from build123d import *

# Parameters (mm, degrees)
SKETCH1_R               = 14.8
BOSS_EXTRUDE1_DEPTH     = 14
SKETCH2_R               = 1.2
CUT_EXTRUDE1_DEPTH      = 1
CUT_EXTRUDE1_DEPTH_BACK = 15
SKETCH3_R               = 5.5
CUT_EXTRUDE2_DEPTH      = 14
CUT_EXTRUDE3_START      = -9
SKETCH5_R               = 2.5
CUT_EXTRUDE3_DEPTH      = 6


with BuildPart() as part:
    # Sketch1 → Boss-Extrude1 (new body)
    with BuildSketch(Plane(origin=(0, 0, 0), x_dir=(0, 0, -1), z_dir=(1, 0, 0))):
        Circle(SKETCH1_R)
    extrude(amount=BOSS_EXTRUDE1_DEPTH)

    # Sketch2 → Cut-Extrude1 (cut, two sides)
    with BuildSketch(Plane(origin=(14, 0, 0), x_dir=(0, 0, -1), z_dir=(1, 0, 0))) as cut_extrude1_sk:
        with Locations((0, 11)):
            Circle(SKETCH2_R)
        with Locations((7.778174593, 7.778174593)):
            Circle(SKETCH2_R)
        with Locations((11, 0)):
            Circle(SKETCH2_R)
        with Locations((7.778174593, -7.778174593)):
            Circle(SKETCH2_R)
        with Locations((0, -11)):
            Circle(SKETCH2_R)
        with Locations((-7.778174593, -7.778174593)):
            Circle(SKETCH2_R)
        with Locations((-11, 0)):
            Circle(SKETCH2_R)
        with Locations((-7.778174593, 7.778174593)):
            Circle(SKETCH2_R)
    extrude(amount=CUT_EXTRUDE1_DEPTH, mode=Mode.SUBTRACT)
    extrude(cut_extrude1_sk.sketch, amount=-CUT_EXTRUDE1_DEPTH_BACK, mode=Mode.SUBTRACT)

    # Sketch3 → Cut-Extrude2 (cut)
    with BuildSketch(Plane.ZY):
        Circle(SKETCH3_R)
    extrude(amount=-CUT_EXTRUDE2_DEPTH, mode=Mode.SUBTRACT)

    # Sketch5 → Cut-Extrude3 (cut, through all)
    with BuildSketch(Plane(origin=(14, 0, 0), x_dir=(0, 0, -1), z_dir=(1, 0, 0)).offset(CUT_EXTRUDE3_START)):
        with Locations((7.778174593, 7.778174593)):
            Circle(SKETCH5_R)
        with Locations((-7.778174593, -7.778174593)):
            Circle(SKETCH5_R)
        with Locations((7.778174593, -7.778174593)):
            Circle(SKETCH5_R)
        with Locations((-7.778174593, 7.778174593)):
            Circle(SKETCH5_R)
    extrude(amount=-CUT_EXTRUDE3_DEPTH, mode=Mode.SUBTRACT)


solid = part.part
Can you work these out from the model? Positions are in its coordinate system, mm. A direction names the side the tool comes from. Coordinates: 2 decimals unless noted, no trailing zeros. Loops run counter-clockwise (first coordinate to the right, second up) from the corner with the lowest first, then second, coordinate; pieces in that order, holes last. Notation, with made-up numbers: (61, -3.5) - (89, -3.5) arc R15 cw to (89, 21.5) - close; hole circle Ø9 at (-9.75, 3.25). An arc over 180 degrees is marked (long way). Answer as a JSON object with one key per item and string values. Group by question number.
Item 1: For pin 1 (14.5 mm diameter, centred on y = 0, z = 0, fed in from +X); pin 2 (3 mm diameter, centred on x = 8, y = 2, fed in from -Z); pin 3 (3 mm diameter, centred on y = -7.78, z = 7.78, fed in from -X); pin 4 (1.5 mm diameter, centred on x = 8.5, y = 3.5, fed in from -Z), each with a flat end and sliding along its axis, tell me the tip position at first contact or that it passes through.
Item 2: If we mould it in two halves opening along Y, with no side actions, what happens to faces 3 (the face through (7.098, 0.36, 9.855)), 4 (the face through (7.1, -12.17, 0.26)), 5 (the face through (6.902, -14.448, 3.208)), 6 (the face through (0, -6, 0))? For each: released by +Y, released by -Y, zero draft, split by the parting line, or undercut.
Item 3: If we section it at C-C (z = -8): List the corners of the cut face in (x, y) for me, plus the area to 3 significant figures.
Item 4: If I drill on L1, parallel to Y at x = 6, z = 0; L2, parallel to Z at x = 2.25, y = -1; L3, parallel to Z at x = 5.5, y = 0.75, over which ranges is the centre line in solid material (lowest first)? Write a range as from..to.
Item 5: If we section it at A-A (y = 0): List the corners of the cut face in (x, z) for me, plus the area to 3 significant figures.
Item 6: On a 3-axis mill with a long thin cutter (end or side, diameter ignored), from which of +Z, -Z, +X, -X, +Y, -Y can I reach the whole of each face in a straight line? I mean faces 1 (the face through (2.54, -9.3, 9.76)), 2 (the face through (14, -6, 0)). Say none if no direction works.
Item 7: If we section it at D-D (x = 4.25): State how many separate pieces and enclosed holes the cut face has, plus the area to 3 significant figures.
Returned:
{
 "1": {"pin 1": "stops at x = 14", "pin 2": "stops at z = -14.79", "pin 3": "stops at x = 5", "pin 4": "stops at z = -14.54"},
 "2": {"face 3": "undercut", "face 4": "undercut", "face 5": "split by the parting line", "face 6": "zero draft"},
 "3": {"outline": "(0, -12.45) - (14, -12.45) - (14, -8.96) - (5, -8.96) - (5, -10.27) - (0, -10.27) - close; (0, -5.29) - (5, -5.29) - (5, -6.6) - (14, -6.6) - (14, 6.6) - (5, 6.6) - (5, 5.29) - (0, 5.29) - close; (0, 10.27) - (5, 10.27) - (5, 8.96) - (14, 8.96) - (14, 12.45) - (0, 12.45) - close", "area": "256 mm²"},
 "4": {"L1": "y = -14.8..-12.2, -9.8..-5.5, 5.5..9.8, 12.2..14.8", "L2": "z = -14.77..-11.66, -10.34..-5.41, 5.41..10.34, 11.66..14.77", "L3": "z = -14.78..-11.94, -10.06..-5.45, 5.45..10.06, 11.94..14.78"},
 "5": {"outline": "(0, -14.8) - (14, -14.8) - (14, -12.2) - (0, -12.2) - close; (0, -9.8) - (14, -9.8) - (14, -5.5) - (0, -5.5) - close; (0, 5.5) - (14, 5.5) - (14, 9.8) - (0, 9.8) - close; (0, 12.2) - (14, 12.2) - (14, 14.8) - (0, 14.8) - close", "area": "193 mm²"},
 "6": {"face 1": "-X", "face 2": "+Z, -Z, +X, +Y, -Y"},
 "7": {"separate pieces": "1", "enclosed holes": "9", "area": "496 mm²"}
}
